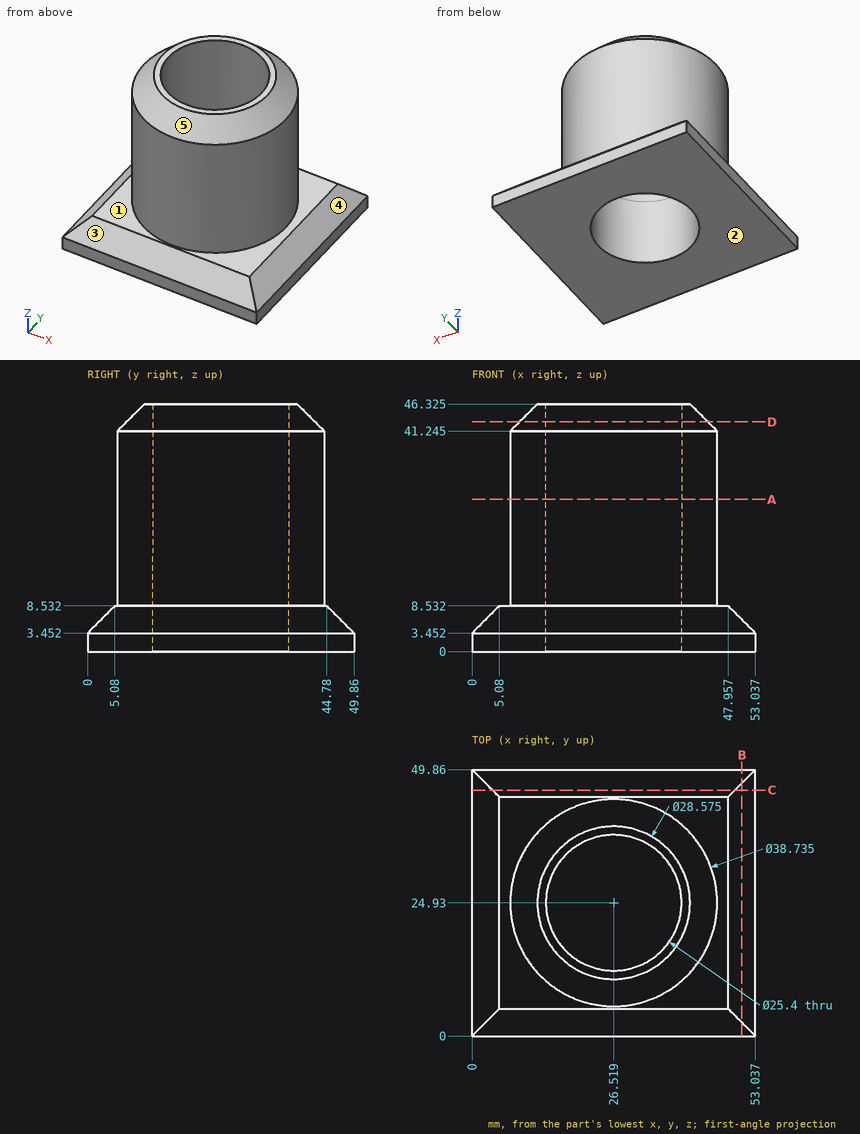
The drawing under review shows one solid part. Ordinate dimensions are in mm from its lowest x, y, z. A direction names the side the tool comes from. Give positions to 0.01 mm unless a question says otherwise; leave off trailing zeros. Write each loop counter-clockwise with the first axis right and the second up, starting at its lowest first coordinate (ties: lowest second). Pieces come first, ordered by that corner, then holes.
1. Draft analysis for pull direction X (two halves, no side actions). For the marked faces 3, 4 and 5, state which applies: +X half, -X half, draft (parallel to the pull), parting line (faces both ways), or undercut.
2. Add section A-A, the plane z = 28.5. Write out the cut boundary in (x, y) (1 decimal), plus the area to 3 significant figures.
3. Add section B-B, the plane x = 50.5. Write out the cut boundary in (y, z), plus the area to 3 significant figures.
4. Add section D-D, the plane z = 43. Write out the cut boundary in (x, y) (1 decimal).
5. Wall thickness on L1, parallel to Z at x = 44, y = 39; L2, parallel to X at y = 35, z = 42 (1 decimal); L3, parallel to Y at x = 31, z = 20.5: over which ranges is each line inside the solid? List them lowest first.
6. Tool access review of the marked faces 1 and 2: name each direction out of +Z, -Z, +X, -X, +Y, -Y from which nothing blocks a thin tool from reaching the whole face with its end or side.
7. For P1, Ø4, axis at x = 20, z = 25.5, coming from the +Y side; P2, Ø3, axis at y = 37.5, z = 17, coming from the -X side; P3, Ø20.5, axis at x = 26.52, y = 24.93, coming from the -Z side; P4, Ø6, axis at x = 41, z = 40, coming from the -Y side, all flat-tipped, find the tip position at first contact; note any pin that passes through.
8. Add section C-C, the plane y = 46. Write out the cut boundary in (x, z), plus the area to 3 significant figures.
Worked answers:
1. face 3: draft
1. face 4: +X half
1. face 5: parting line
2. outline: circle Ø38.7 at (26.5, 24.9); hole circle Ø25.4 at (26.5, 24.9)
2. area: 672 mm2
3. outline: (0, 0) - (49.86, 0) - (49.86, 3.45) - (47.32, 5.99) - (2.54, 5.99) - (0, 3.45) - close
3. area: 292 mm2
4. outline: circle Ø35.2 at (26.5, 24.9); hole circle Ø25.4 at (26.5, 24.9)
5. L1: z = 0 to 8.53
5. L2: x = 10.9 to 18.8, 34.3 to 42.2
5. L3: y = 6.09 to 13.05, 36.81 to 43.77
6. face 1: +Z
6. face 2: -Z, +X, -X, +Y, -Y
7. P1: stops at y = 43.76
7. P2: stops at x = 10.63
7. P3: passes through
7. P4: stops at y = 9.33
8. outline: (0, 0) - (53.04, 0) - (53.04, 3.45) - (49.18, 7.31) - (3.86, 7.31) - (0, 3.45) - close
8. area: 373 mm2
